Here's how the part is built. I have some questions about the finished solid (model axes, mm). A direction names the side the tool comes from. Coordinates: 2 decimals unless noted, no trailing zeros. Write each loop counter-clockwise with the first axis right and the second up, starting at its lowest first coordinate (ties: lowest second). Pieces come first, ordered by that corner, then holes. Notation, with made-up numbers: (59.25, 5) -> (87.25, 5) arc R20 cw to (87.25, 35) -> close; hole circle Ø3 at (24.5, 66.25). An arc over 180 degrees is marked (long way). Use a Markdown table: item, result. Add a question column.
Item 1: On a 3-axis mill with a long thin cutter (end or side, diameter ignored), from which of +Z, -Z, +X, -X, +Y, -Y can I reach the whole of each face in a straight line? I mean faces 1 (the flat face through (0, -1.4, 3)), 2 (the cylindrical face through (5.465, 0.006, 0.301)). Say none if no direction works.
Item 2: If I drill on line 1 along Y through (x, z) = (0.5, 3.75); line 2 along X through (y, z) = (0, 6), over which ranges is the centre line in solid material (lowest first)? Write a range as from..to.
Item 3: Imagine slicing it at C-C, the plane z = 0.75. Write out the boundary of the cut face in (x, y), and give its area (3 significant figures).
Item 4: Imagine slicing it at B-B, the plane z = 3.5. Write out the boundary of the cut face in (x, y), and give its area (3 significant figures).
Item 5: If we mould it in two halves opening along Y, with no side actions, what happens to faces 3 (the cylindrical face through (5.15, -1.83, 3.46)), 4 (the cylindrical face through (4.465, -1.099, 3.451)), 5 (the cylindrical face through (-0.053, 2.115, 0.301))? For each: pulls with the +Y half, pulls with the -Y half, needs draft (parallel to the pull), parting line crosses it, or undercut.
```python
from build123d import *

# Parameters (mm, degrees)
F1_DEPTH = 7
F2_R     = 0.99999


# Not quite as in the source:
# - a fillet or chamfer is up to 0.001 mm smaller than in the source, because OpenCascade refuses the exact size


with BuildPart() as f1:
    # F0 (on Top) → F1 (new body)
    with BuildSketch(Plane.XY):
        with BuildLine():
            Line((-3.75, -2.4), (3.75, -2.4))
            ThreePointArc((3.75, -2.4), (5.1642135624, -1.8142135624), (5.75, -0.4))
            Line((5.75, -0.4), (5.75, 0.4))
            ThreePointArc((5.75, 0.4), (5.1642135624, 1.8142135624), (3.75, 2.4))
            Line((3.75, 2.4), (-3.75, 2.4))
            ThreePointArc((-3.75, 2.4), (-5.1642135624, 1.8142135624), (-5.75, 0.4))
            Line((-5.75, 0.4), (-5.75, -0.4))
            ThreePointArc((-5.75, -0.4), (-5.1642135624, -1.8142135624), (-3.75, -2.4))
        make_face()
        with BuildLine():
            ThreePointArc((4.75, -0.4), (4.4571067812, -1.1071067812), (3.75, -1.4))
            Line((3.75, -1.4), (-3.75, -1.4))
            ThreePointArc((-3.75, -1.4), (-4.4571067812, -1.1071067812), (-4.75, -0.4))
            Line((-4.75, -0.4), (-4.75, 0.4))
            ThreePointArc((-4.75, 0.4), (-4.4571067812, 1.1071067812), (-3.75, 1.4))
            Line((-3.75, 1.4), (3.75, 1.4))
            ThreePointArc((3.75, 1.4), (4.4571067812, 1.1071067812), (4.75, 0.4))
            Line((4.75, 0.4), (4.75, -0.4))
        make_face(mode=Mode.SUBTRACT)
    extrude(amount=F1_DEPTH)

    # F2 (radius 1 in the source; OpenCascade refuses exactly that, so slightly less here)
    f2_edges = [f1.edges().sort_by_distance(p)[0] for p in [
        (0, 2.4, 7),
        (0, 2.4, 0),
    ]]
    fillet(f2_edges, radius=F2_R)


solid = f1.part
```
Ans:
| question | item | result |
|---|---|---|
| 1 | face 1 | +Z, -Z |
| 1 | face 2 | -Z, +X, +Y, -Y |
| 2 | line 1 | y = -2.4..-1.4, 1.4..2.4 |
| 2 | line 2 | x = -5.75..-4.75, 4.75..5.75 |
| 3 | outline | (-5.72, -0.4) arc R1.97 ccw to (-3.75, -2.37) -> (3.75, -2.37) arc R1.97 ccw to (5.72, -0.4) -> (5.72, 0.4) arc R1.97 ccw to (3.75, 2.37) -> (-3.75, 2.37) arc R1.97 ccw to (-5.72, 0.4) -> close; hole (-4.75, -0.4) arc R1 ccw to (-3.75, -1.4) -> (3.75, -1.4) arc R1 ccw to (4.75, -0.4) -> (4.75, 0.4) arc R1 ccw to (3.75, 1.4) -> (-3.75, 1.4) arc R1 ccw to (-4.75, 0.4) -> close |
| 3 | area | 25.1 mm^2 |
| 4 | outline | (-5.75, -0.4) arc R2 ccw to (-3.75, -2.4) -> (3.75, -2.4) arc R2 ccw to (5.75, -0.4) -> (5.75, 0.4) arc R2 ccw to (3.75, 2.4) -> (-3.75, 2.4) arc R2 ccw to (-5.75, 0.4) -> close; hole (-4.75, -0.4) arc R1 ccw to (-3.75, -1.4) -> (3.75, -1.4) arc R1 ccw to (4.75, -0.4) -> (4.75, 0.4) arc R1 ccw to (3.75, 1.4) -> (-3.75, 1.4) arc R1 ccw to (-4.75, 0.4) -> close |
| 4 | area | 26.0 mm^2 |
| 5 | face 3 | pulls with the -Y half |
| 5 | face 4 | undercut |
| 5 | face 5 | pulls with the +Y half |
